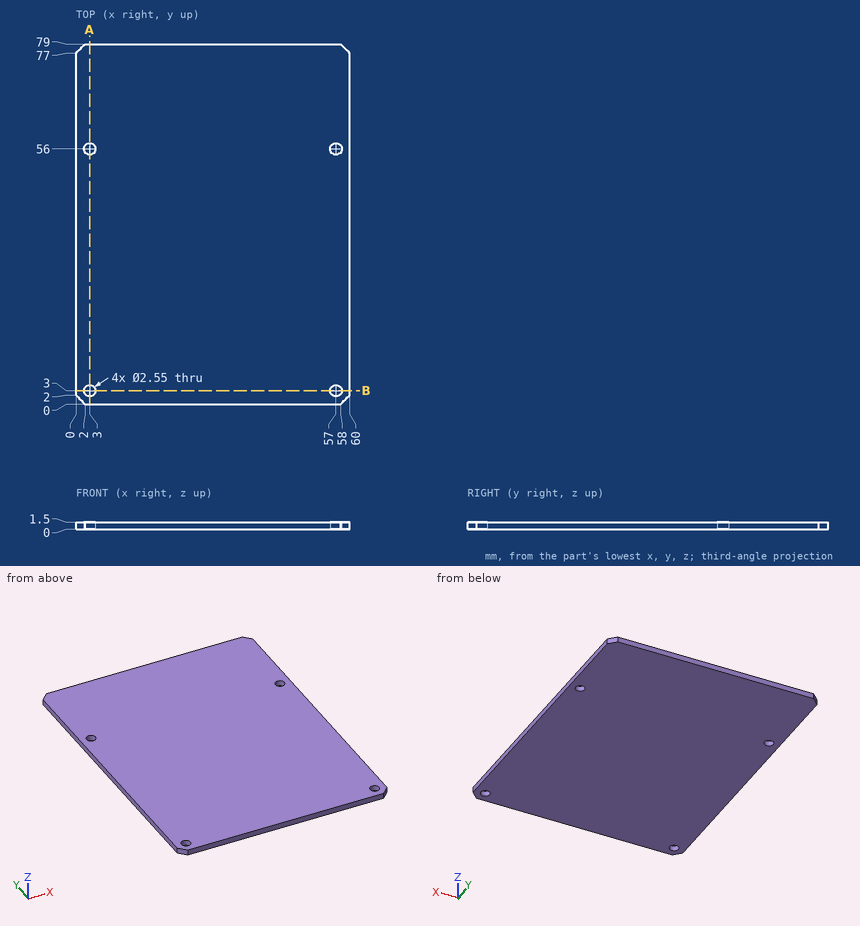
Job drawing, mm, ordinate dimensions from the low corner. One solid piece. Coordinates: 2 decimals unless noted, no trailing zeros. Write each loop counter-clockwise with the first axis right and the second up, starting at its lowest first coordinate (ties: lowest second). Pieces come first, ordered by that corner, then holes. Notation, with made-up numbers: M 19.5,30.5 L 71.5,30.5 A23 cw 71.5,48.5 Z; hole C -6.75,-22 d10. An arc over 180 degrees is marked long. Answer as a JSON object with one key per item and string values. Group by question number.
1) Wall check: line 1 (Y direction, x = 57, z = 0.9) (3 decimals). Give the ranges that are in metal, low to high. Write a range as from..to.
2) Saw through at A-A (x = 3). Write the cut outline in (y, z) (3 decimals).
3) Saw through at B-B (y = 3). Write the cut outline in (x, z) (3 decimals), plus the area to 4 significant figures.
4) Pin check, flat tip, straight feed: pin 1 Ø1.5 at (x, y) = (57, 56) entering from -Z. Stop position of the tip, or through.
Values follow:
{
 "1": {"line 1": "y = 0..1.725, 4.275..54.725, 57.275..79"},
 "2": {"outline": "M 0,0 L 1.725,0 L 1.725,1.5 L 0,1.5 Z; M 4.275,0 L 54.725,0 L 54.725,1.5 L 4.275,1.5 Z; M 57.275,0 L 79,0 L 79,1.5 L 57.275,1.5 Z"},
 "3": {"outline": "M 0,0 L 1.725,0 L 1.725,1.5 L 0,1.5 Z; M 4.275,0 L 55.725,0 L 55.725,1.5 L 4.275,1.5 Z; M 58.275,0 L 60,0 L 60,1.5 L 58.275,1.5 Z", "area": "82.35 mm2"},
 "4": {"pin 1": "passes through"}
}
